For this review, take the finished solid that the model builds, in its own axes (mm). Face numbers are marked on the shaded views. Coordinates: 2 decimals unless noted, no trailing zeros. Loops run counter-clockwise (first coordinate to the right, second up) from the corner with the lowest first, then second, coordinate; pieces in that order, holes last. Notation, with made-up numbers: (0, 13) - (8, 13) arc R17 cw to (8, 21) - close; hole circle Ø3 at (-15, 82.5). An arc over 180 degrees is marked (long way). Use one line per item in the form item = value. Start each with the question number.
1. Add section C-C on y = 25.5. Give the boundary of the cut face in (x, z) (3 decimals).
2. For pin 1 Ø3.5 at (x, z) = (-17.5, -13.5) entering from -Y (3 decimals); pin 2 Ø12 at (x, z) = (-13, 2) entering from -Y; pin 3 Ø4 at (y, z) = (9, 9) entering from -X; pin 4 Ø4 at (x, y) = (10.5, 24.5) entering from -Z, all flat-tipped, find the tip position at first contact; note any pin that passes through.
3. Draft analysis for pull direction Z (two halves, no side actions). For the marked faces 1, 2 and 3, state which applies: +Z half, -Z half, draft (parallel to the pull), parting line (faces both ways), or undercut.
4. Add section A-A on x = 0. Count the separate pieces of the cut face and the enclosed holes in it, and give its area (3 significant figures).
5. Add section B-B on z = 0. Give the boundary of the cut face in (x, y) (3 decimals).
6. To check wall thickness, follow probe 1 along Y at (x, z) = (-11, -11) (3 decimals); probe 2 along X at (y, z) = (42, -7.5); probe 3 along Z at (x, y) = (1.5, 25.5). State the ranges of each line that lie inside material, in increasing order.
7. Add section D-D on x = -12. Give the boundary of the cut face in (y, z) (3 decimals), and give its area (3 significant figures).
```python
from build123d import *

# Parameters (mm, degrees)
SKETCH1_R                = 20.32
BOSS_EXTRUDE1_DEPTH      = 50.8
SHELL1_T                 = -3.175
CUT_EXTRUDE1_DEPTH       = 56.623245366
CUT_EXTRUDE1_DEPTH_BACK  = 46.482
SKETCH2_R                = 4.064
BOSS_EXTRUDE2_START      = -34.925
BOSS_EXTRUDE2_DEPTH      = 12.7
SKETCH4_R                = 1.5875
CUT_EXTRUDE2_DEPTH       = 19.05
FILLET1_R                = 6.35
CIRPATTERN1_COUNT        = 3
FILLET1_OF_CIRPATTERN1_R = 6.35


with BuildPart() as part:
    # Sketch1 → Boss-Extrude1 (new body)
    with BuildSketch(Plane(origin=(0, 0, 0), x_dir=(1, 0, 0), z_dir=(0, 1, 0))):
        with Locations(Location((0, 0, 0), (0, 0, 270))):
            Circle(SKETCH1_R)
    extrude(amount=BOSS_EXTRUDE1_DEPTH)

    # Shell1
    shell1_openings = [part.faces().sort_by_distance(p)[0] for p in [
        (0, 50.8, 0),
    ]]
    offset(amount=SHELL1_T, openings=shell1_openings, kind=Kind.INTERSECTION)

    # Sketch2 → Cut-Extrude1 (cut, two sides: drawn at the far end of the back side and taken through both)
    with BuildSketch(Plane(origin=(0, 3.175, 0), x_dir=(1, 0, 0), z_dir=(0, 1, 0)).offset(-CUT_EXTRUDE1_DEPTH_BACK)):
        with Locations(Location((0, 0, 0), (0, 0, 270))):
            Circle(SKETCH2_R)
    extrude(amount=CUT_EXTRUDE1_DEPTH + CUT_EXTRUDE1_DEPTH_BACK, mode=Mode.SUBTRACT)

    # Sketch3 → Boss-Extrude2 (add)
    with BuildSketch(Plane.XZ.offset(BOSS_EXTRUDE2_START)):
        with BuildLine():
            ThreePointArc((-9.525, 17.949283412), (0, 20.32), (9.525, 17.949283412))
            Line((9.525, 17.949283412), (9.525, 26.67))
            Line((9.525, 26.67), (-9.525, 26.67))
            Line((-9.525, 26.67), (-9.525, 17.949283412))
        make_face()
    boss_extrude2 = extrude(amount=-BOSS_EXTRUDE2_DEPTH)

    # Sketch4 → Cut-Extrude2 (cut)
    with BuildSketch(Plane(origin=(9.525, 0, 0), x_dir=(0, 0, -1), z_dir=(1, 0, 0))):
        with Locations((-23.495, 41.275)):
            Circle(SKETCH4_R)
    cut_extrude2 = extrude(amount=-CUT_EXTRUDE2_DEPTH, mode=Mode.SUBTRACT)

    # Fillet1
    fillet1_edges = [part.edges().sort_by_distance(p)[0] for p in [
        (0, 47.625, 26.67),
        (0, 34.925, 26.67),
    ]]
    fillet(fillet1_edges, radius=FILLET1_R - 0.0001)  # a hair under: the kernel refuses the full size

    # CirPattern1: Boss-Extrude2, Cut-Extrude2 ×3 about axis
    cirpattern1_axis = Axis((0, 0, 0), (0, 1, 0))
    add([boss_extrude2.rotate(cirpattern1_axis, i * 360 / CIRPATTERN1_COUNT) for i in range(1, CIRPATTERN1_COUNT)])
    add([cut_extrude2.rotate(cirpattern1_axis, i * 360 / CIRPATTERN1_COUNT) for i in range(1, CIRPATTERN1_COUNT)], mode=Mode.SUBTRACT)

    # Fillet1 of CirPattern1
    fillet1_of_cirpattern1_edges = [part.edges().sort_by_distance(p)[0] for p in [
        (23.096897519, 47.625, -13.335),
        (23.096897519, 34.925, -13.335),
        (-23.096897519, 47.625, -13.335),
        (-23.096897519, 34.925, -13.335),
    ]]
    fillet(fillet1_of_cirpattern1_edges, radius=FILLET1_OF_CIRPATTERN1_R - 0.0001)  # a hair under: the kernel refuses the full size


solid = part.part
```
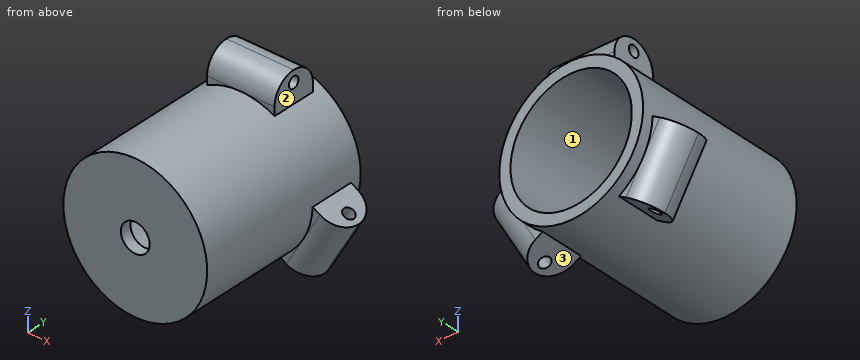
Conclusion:
q1.outline = circle Ø40.64 at (0, 0); hole circle Ø34.29 at (0, 0)
q2.pin_1 = 34.925
q2.pin_2 = 0
q2.pin_3 = -19.08
q2.pin_4 = -18.46
q3.face_1 = undercut
q3.face_2 = draft
q3.face_3 = -Z half
q4.separate_pieces = 2
q4.enclosed_holes = 1
q4.area = 461 mm^2
q5.outline = (-20.32, 0) - (-4.064, 0) - (-4.064, 3.175) - (-17.145, 3.175) - (-17.145, 50.8) - (-20.32, 50.8) - close; (4.064, 0) - (20.32, 0) - (20.32, 50.8) - (17.145, 50.8) - (17.145, 3.175) - (4.064, 3.175) - close
q6.probe_1 = 0 to 3.175
q6.probe_2 = -26.42 to -24.43, -21.17 to -15.42, 15.42 to 21.17, 24.43 to 26.42
q6.probe_3 = -20.26 to -17.08, 17.08 to 20.26
q7.outline = (0, -16.398) - (34.925, -16.398) - (34.925, -17.927) - (47.625, -17.927) - (47.625, -16.398) - (50.8, -16.398) - (50.8, -12.245) - (3.175, -12.245) - (3.175, 12.245) - (50.8, 12.245) - (50.8, 16.398) - (0, 16.398) - close
q7.area = 519 mm^2
